from build123d import *

# Parameters (mm, degrees)
SKETCH1_W           = 23.8
SKETCH1_H           = 3.2
BOSS_EXTRUDE1_DEPTH = 7.8
SHELL1_T            = -1.2
SKETCH3_R           = 1.5
SKETCH3_R_2         = 0.6
BOSS_EXTRUDE3_DEPTH = 1.8
LPATTERN1_COUNT     = 2
LPATTERN1_PITCH     = 8
BOSS_EXTRUDE4_DEPTH = 1.5


with BuildPart() as part:
    # Sketch1 → Boss-Extrude1 (new body)
    with BuildSketch(Plane.XY):
        with Locations((11.9, 1.6)):
            Rectangle(SKETCH1_W, SKETCH1_H)
    extrude(amount=-BOSS_EXTRUDE1_DEPTH)

    # Shell1
    shell1_openings = [part.faces().sort_by_distance(p)[0] for p in [
        (11.9, 0, -3.9),
    ]]
    offset(amount=SHELL1_T, openings=shell1_openings, kind=Kind.INTERSECTION)

    # Sketch3 → Boss-Extrude3 (add)
    with BuildSketch(Plane.XZ.offset(-2)):
        with Locations(Location((15.9, -3.9, 0), (0, 0, 90))):
            Circle(SKETCH3_R)
        with Locations(Location((15.9, -3.9, 0), (0, 0, 270))):
            Circle(SKETCH3_R_2, mode=Mode.SUBTRACT)
    boss_extrude3 = extrude(amount=BOSS_EXTRUDE3_DEPTH)

    # LPattern1: Boss-Extrude3 ×2
    with Locations(*[(-i * LPATTERN1_PITCH, 0, 0) for i in range(1, LPATTERN1_COUNT)]):
        add(boss_extrude3)

    # Sketch4 → Boss-Extrude4 (add)
    with BuildSketch(Plane(origin=(0, 0, -7.8), x_dir=(-1, 0, 0), z_dir=(0, 0, -1))):
        Polygon((-23.8, 3.2), (-23.8, 9.6), (0, 9.6), (0, 3.2), (0, 0), (-23.8, 0), align=None)
    extrude(amount=-BOSS_EXTRUDE4_DEPTH)


solid = part.part
Model file for the job. Use its own axes, mm. A direction names the side the tool comes from. Give positions to 0.01 mm unless a question says otherwise; leave off trailing zeros. Loops run counter-clockwise (first coordinate to the right, second up) from the corner with the lowest first, then second, coordinate; pieces in that order, holes last.
Item 1: Slice it at A-A (z = -3). Write the cut outline in (x, y), plus the area to 3 significant figures.
Check values:
outline: (0, 0) - (1.2, 0) - (1.2, 2) - (6.7, 2) - (6.7, 0.2) - (9.1, 0.2) - (9.1, 2) - (14.7, 2) - (14.7, 0.2) - (17.1, 0.2) - (17.1, 2) - (22.6, 2) - (22.6, 0) - (23.8, 0) - (23.8, 3.2) - (0, 3.2) - close
area: 42.0 mm2
Item 2: Mould opens along X. For faces 4 (the face through (23.8, 3, -5)), 5 (the face through (12, 9.6, -7)), 6 (the face through (15.37, 1.11, -4.18)), 7 (the face through (12, 1, -6.3)) say: +X half, -X half, draft (parallel to the pull), parting line (faces both ways), or undercut.
Check values:
face 4: +X half
face 5: draft
face 6: undercut
face 7: undercut
Item 3: Drill centre lines: line 1 along X through (y, z) = (1.45, -3.9); line 2 along Z through (x, y) = (6.25, 4.75); line 3 along Y through (x, z) = (20.5, -2.5). Where is each one in solid material? Low to high.
Check values:
line 1: x = 0 to 1.2, 6.4 to 7.3, 8.5 to 9.4, 14.4 to 15.3, 16.5 to 17.4, 22.6 to 23.8
line 2: z = -7.8 to -6.3
line 3: y = 2 to 3.2
Item 4: Slice it at D-D (x = 7.9). Write the cut outline in (y, z), plus the area to 3 significant figures.
Check values:
outline: (0, -7.8) - (9.6, -7.8) - (9.6, -6.3) - (3.2, -6.3) - (3.2, 0) - (0, 0) - (0, -1.2) - (2, -1.2) - (2, -2.4) - (0.2, -2.4) - (0.2, -3.3) - (2, -3.3) - (2, -4.5) - (0.2, -4.5) - (0.2, -5.4) - (2, -5.4) - (2, -6.3) - (0, -6.3) - close
area: 27.6 mm2
Item 5: Drop flat-ended pins along their axis: P1, Ø3, axis at x = 14.5, z = -1.5, coming from the +Y side; P2, Ø3.5, axis at x = 16, z = -4, coming from the -Y side; P3, Ø1.9, axis at x = 16, y = 6.5, coming from the +Z side. Give the stop position or say it passes through.
Check values:
P1: stops at y = 3.2
P2: stops at y = 0.2
P3: stops at z = -6.3
Item 6: Slice it at C-C (y = 4). Write the cut outline in (x, z).
Check values:
outline: (0, -7.8) - (23.8, -7.8) - (23.8, -6.3) - (0, -6.3) - close
Item 7: Which spindle directions (+Z, -Z, +X, -X, +Y, -Y) get a long thin tool onto all of the face, cutting with end or side? Do faces 1 (the face through (12, 5, -7.8)), 2 (the face through (8.08, 1.113, -4.472)), 3 (the face through (12, 6, -6.3)). Say none if no direction does.
Check values:
face 1: -Z, +X, -X, +Y, -Y
face 2: -Y
face 3: +Z, +X, -X, +Y
Item 8: Slice it at B-B (x = 20). Write the cut outline in (y, z), plus the area to 3 significant figures.
Check values:
outline: (0, -7.8) - (9.6, -7.8) - (9.6, -6.3) - (3.2, -6.3) - (3.2, 0) - (0, 0) - (0, -1.2) - (2, -1.2) - (2, -6.3) - (0, -6.3) - close
area: 24.4 mm2
